For this review, take the finished solid that the model builds, in its own axes (mm). A direction names the side the tool comes from. Coordinates: 2 decimals unless noted, no trailing zeros. Write each loop counter-clockwise with the first axis right and the second up, starting at its lowest first coordinate (ties: lowest second). Pieces come first, ordered by that corner, then holes. Notation, with made-up numbers: M 35,-2 L 75,-2 A21 cw 75,12 Z; hole C 47.25,38 d2. An arc over 180 degrees is marked long. One line per question, with ' | ' between items.
from build123d import *

# Parameters (mm, degrees)
CYLINDER014_R     = 5.75
CYLINDER014_DEPTH = 10
CYLINDER013_R     = 3
CYLINDER013_DEPTH = 10


with BuildPart() as obj1:
    # Cylinder014 → Cylinder014 (new body)
    with BuildSketch(Plane(origin=(-23, 0, 69), x_dir=(1, 0, 0), z_dir=(0, 0, 1))):
        Circle(CYLINDER014_R)
    extrude(amount=CYLINDER014_DEPTH)


with BuildPart() as fusion003:
    # Cylinder013 → Cylinder013 (new body)
    with BuildSketch(Plane(origin=(-23, 0, 65), x_dir=(1, 0, 0), z_dir=(0, 0, 1))):
        Circle(CYLINDER013_R)
    extrude(amount=CYLINDER013_DEPTH)

    # Fusion003: union obj1
    add(obj1.part)


with BuildPart() as fusion003_1:
    # Fusion003 placement: moved
    add(fusion003.part.moved(Location((2.5, -25, -6))))


solid = fusion003_1.part
1. Machinability: for faces 1 (the flat face through (-21, -25, 73)), 2 (the flat face through (-18, -27, 63)), which of the approach directions +Z, -Z, +X, -X, +Y, -Y give a long, thin tool a straight path to every point of the face, cutting with its end or side? Answer none if there is none.
Computed values:
face 1: +Z, +X, -X, +Y, -Y | face 2: -Z
2. Take a section at A-A on y = -25. State the section outline as (x, z) points, plus the area to 3 significant figures.
Computed values:
outline: M -26.25,63 L -23.5,63 L -23.5,59 L -17.5,59 L -17.5,63 L -14.75,63 L -14.75,73 L -26.25,73 Z | area: 139 mm2
3. For line 1 along Z through (x, y) = (-24.25, -27.75); line 2 along X through (y, z) = (-29.75, 71); line 3 along X through (y, z) = (-25.75, 60.25), list the stretches that pass through material, from the lowest coordinate up.
Computed values:
line 1: z = 63 to 73 | line 2: x = -23.74 to -17.26 | line 3: x = -23.4 to -17.6
4. Take a section at D-D on z = 60.5. State the section outline as (x, y) points, plus the area to 3 significant figures.
Computed values:
outline: C -20.5,-25 d6 | area: 28.3 mm2
5. Take a section at C-C on z = 71.25. State the section outline as (x, y) points, plus the area to 3 significant figures.
Computed values:
outline: C -20.5,-25 d11.5 | area: 104 mm2
6. Clearance check with flat-ended pins moving along their axes: P1, Ø1.5, axis at x = -24, z = 71, coming from the -Y side; P2, Ø4, axis at x = -21.5, z = 60.5, coming from the +Y side; P3, Ø5, axis at y = -21, z = 71, coming from the +X side. State where each tip first meets the part, or that it passes through.
Computed values:
P1: stops at y = -30.05 | P2: stops at y = -22 | P3: stops at x = -14.95
7. Take a section at B-B on x = -20.5. State the section outline as (y, z) points.
Computed values:
outline: M -30.75,63 L -28,63 L -28,59 L -22,59 L -22,63 L -19.25,63 L -19.25,73 L -30.75,73 Z
